Design review of the part built by this model. Coordinates are the model's own, in mm. A direction names the side the tool comes from. Coordinates: 2 decimals unless noted, no trailing zeros. Loops run counter-clockwise (first coordinate to the right, second up) from the corner with the lowest first, then second, coordinate; pieces in that order, holes last. Notation, with made-up numbers: M -36.5,22.5 L -16.5,22.5 A9 cw -16.5,38.5 Z; hole C 7.5,-21 d3. An arc over 180 degrees is marked long. Answer as CSV lines item,"result". Start each with the question number.
from build123d import *

# Parameters (mm, degrees)
SKETCH_1_W      = 90
SKETCH_1_H      = 100
SKETCH_1_R      = 6.372546474
SKETCH_1_R_2    = 2
SKETCH_1_R_3    = 1.5
SKETCH_1_W_2    = 4.4
SKETCH_1_H_2    = 8.4
EXTRUDE_1_DEPTH = 4


with BuildPart() as part:
    # 草图1 → 凸台-拉伸1 (new body)
    with BuildSketch(Plane.XY):
        Rectangle(SKETCH_1_W, SKETCH_1_H)
        Circle(SKETCH_1_R, mode=Mode.SUBTRACT)
        with Locations((0, -19)):
            Circle(SKETCH_1_R_2, mode=Mode.SUBTRACT)
        with Locations((-13.435028843, -13.435028843)):
            Circle(SKETCH_1_R_2, mode=Mode.SUBTRACT)
        with Locations((-19, 0)):
            Circle(SKETCH_1_R_2, mode=Mode.SUBTRACT)
        with Locations((-13.435028843, 13.435028843)):
            Circle(SKETCH_1_R_2, mode=Mode.SUBTRACT)
        with Locations((0, 19)):
            Circle(SKETCH_1_R_2, mode=Mode.SUBTRACT)
        with Locations((13.435028843, 13.435028843)):
            Circle(SKETCH_1_R_2, mode=Mode.SUBTRACT)
        with Locations((19, 0)):
            Circle(SKETCH_1_R_2, mode=Mode.SUBTRACT)
        with Locations((13.435028843, -13.435028843)):
            Circle(SKETCH_1_R_2, mode=Mode.SUBTRACT)
        with Locations((-20, -40)):
            Circle(SKETCH_1_R_2, mode=Mode.SUBTRACT)
        with Locations((20, -40)):
            Circle(SKETCH_1_R_2, mode=Mode.SUBTRACT)
        with Locations(Location((20, 40, 0), (0, 0, 180))):
            Circle(SKETCH_1_R_2, mode=Mode.SUBTRACT)
        with Locations(Location((-20, 40, 0), (0, 0, 180))):
            Circle(SKETCH_1_R_2, mode=Mode.SUBTRACT)
        with Locations((37, 0)):
            Circle(SKETCH_1_R_3, mode=Mode.SUBTRACT)
        with Locations((37, 26)):
            Circle(SKETCH_1_R_3, mode=Mode.SUBTRACT)
        with Locations(Location((37, -26, 0), (0, 0, 180))):
            Circle(SKETCH_1_R_3, mode=Mode.SUBTRACT)
        with Locations(Location((-37, 0, 0), (0, 0, 180))):
            Circle(SKETCH_1_R_3, mode=Mode.SUBTRACT)
        with Locations((-37, -26)):
            Circle(SKETCH_1_R_3, mode=Mode.SUBTRACT)
        with Locations(Location((-37, 26, 0), (0, 0, 180))):
            Circle(SKETCH_1_R_3, mode=Mode.SUBTRACT)
        with Locations((37, -13)):
            Rectangle(SKETCH_1_W_2, SKETCH_1_H_2, mode=Mode.SUBTRACT)
        with Locations((37, 13)):
            Rectangle(SKETCH_1_W_2, SKETCH_1_H_2, mode=Mode.SUBTRACT)
        with Locations((-37, 13)):
            Rectangle(SKETCH_1_W_2, SKETCH_1_H_2, mode=Mode.SUBTRACT)
        with Locations((-37, -13)):
            Rectangle(SKETCH_1_W_2, SKETCH_1_H_2, mode=Mode.SUBTRACT)
    extrude(amount=EXTRUDE_1_DEPTH)


solid = part.part
Item 1: For faces 1 (the face through (9, 1, 0)), 2 (the face through (37, -8.8, 2)), list the 3-axis set-ups (+Z, -Z, +X, -X, +Y, -Y) from which the entire face can be reached by the end or side of a thin tool; tool diameter is ignored.
Item 2: Add section B-B (y = -40). Give the boundary of the cut face in (x, z).
Item 3: Add section D-D (x = -3.5). Give the boundary of the cut face in (y, z), plus the area to 3 significant figures.
Item 4: For pin 1 (2.5 mm diameter, centred on x = -13.44, y = 13.44, fed in from +Z), flat-tipped, find the tip position at first contact; note if it passes through.
Item 5: For line 1 along X through (y, z) = (40, 1.9); line 2 along Y through (x, z) = (-37, 1.4); line 3 along Y through (x, z) = (0, 1.5), list the stretches that pass through material, from the lowest coordinate up. Write a range as from..to.
Item 6: Add section A-A (x = -37). Give the boundary of the cut face in (y, z).
Item 7: Mouldability with a two-part tool opening along X and no side actions: class faces 3 (the face through (45, -1, 2)), 4 (the face through (34.8, -13, 2)), 5 (the face through (-1, 50, 2)) as released by +X, released by -X, zero draft, split by the parting line, or undercut.
Item 8: Add section C-C (y = -19). Give the boundary of the cut face in (x, z), plus the area to 3 significant figures.
Response:
1,face 1,"-Z, +X, -X, +Y, -Y"
1,face 2,"+Z, -Z"
2,outline,"M -45,0 L -22,0 L -22,4 L -45,4 Z; M -18,0 L 18,0 L 18,4 L -18,4 Z; M 22,0 L 45,0 L 45,4 L 22,4 Z"
3,outline,"M -50,0 L -5.33,0 L -5.33,4 L -50,4 Z; M 5.33,0 L 50,0 L 50,4 L 5.33,4 Z"
3,area,"357 mm²"
4,pin 1,"through"
5,line 1,"-45..-22, -18..18, 22..45"
5,line 2,"-50..-27.5, -24.5..-17.2, -8.8..-1.5, 1.5..8.8, 17.2..24.5, 27.5..50"
5,line 3,"-50..-21, -17..-6.37, 6.37..17, 21..50"
6,outline,"M -50,0 L -27.5,0 L -27.5,4 L -50,4 Z; M -24.5,0 L -17.2,0 L -17.2,4 L -24.5,4 Z; M -8.8,0 L -1.5,0 L -1.5,4 L -8.8,4 Z; M 1.5,0 L 8.8,0 L 8.8,4 L 1.5,4 Z; M 17.2,0 L 24.5,0 L 24.5,4 L 17.2,4 Z; M 27.5,0 L 50,0 L 50,4 L 27.5,4 Z"
7,face 3,"released by +X"
7,face 4,"undercut"
7,face 5,"zero draft"
8,outline,"M -45,0 L -2,0 L -2,4 L -45,4 Z; M 2,0 L 45,0 L 45,4 L 2,4 Z"
8,area,"344 mm²"
